Build history of the part. All positions in model axes, mm. Face numbers are marked on the shaded views. A direction names the side the tool comes from. Give positions to 0.01 mm unless a question says otherwise; leave off trailing zeros. Write each loop counter-clockwise with the first axis right and the second up, starting at its lowest first coordinate (ties: lowest second). Pieces come first, ordered by that corner, then holes. Notation, with made-up numbers: (1.25, 7) - (13.25, 7) arc R27 cw to (13.25, 43) - close; hole circle Ø11 at (-32, 48). An arc over 180 degrees is marked (long way). Use one line per item in the form item = value. Start each with the question number.
from build123d import *

# Parameters (mm, degrees)
F1_DEPTH = 6.35
F2_W     = 6
F2_H     = 6
F3_DEPTH = 6.35


# Not quite as in the source:
# - a length typed as a fraction of an inch, garbled in the dataset ("3 / 203.2 mm" for 3/8 in), is restored


with BuildPart() as f1:
    # F0 (on Front) → F1 (new body)
    with BuildSketch(Plane.XZ):
        with BuildLine():
            ThreePointArc((9.85, 6.4062469512), (11.2649900133, 3.3410327745), (11.75, 0))
            ThreePointArc((11.75, 0), (11.2649900133, -3.3410327745), (9.85, -6.4062469512))
            Line((9.85, -6.4062469512), (9.85, -13.5476935306))
            ThreePointArc((9.85, -13.5476935306), (14.9256490646, -7.6018089952), (16.75, 0))
            ThreePointArc((16.75, 0), (14.9256490646, 7.6018089952), (9.85, 13.5476935306))
            Line((9.85, 13.5476935306), (9.85, 6.4062469512))
        make_face()
        with BuildLine():
            ThreePointArc((-9.85, 6.4062469512), (0, 11.75), (9.85, 6.4062469512))
            Line((9.85, 6.4062469512), (9.85, 13.5476935306))
            ThreePointArc((9.85, 13.5476935306), (0, 16.75), (-9.85, 13.5476935306))
            Line((-9.85, 13.5476935306), (-9.85, 6.4062469512))
        make_face()
        with BuildLine():
            Line((9.85, -13.5476935306), (9.85, -6.4062469512))
            ThreePointArc((9.85, -6.4062469512), (0, -11.75), (-9.85, -6.4062469512))
            Line((-9.85, -6.4062469512), (-9.85, -13.5476935306))
            ThreePointArc((-9.85, -13.5476935306), (0, -16.75), (9.85, -13.5476935306))
        make_face()
        with BuildLine():
            ThreePointArc((-9.85, -6.4062469512), (-11.75, 0), (-9.85, 6.4062469512))
            Line((-9.85, 6.4062469512), (-9.85, 13.5476935306))
            ThreePointArc((-9.85, 13.5476935306), (-16.75, 0), (-9.85, -13.5476935306))
            Line((-9.85, -13.5476935306), (-9.85, -6.4062469512))
        make_face()
        with BuildLine():
            ThreePointArc((-9.85, 13.5476935306), (0, 16.75), (9.85, 13.5476935306))
            Line((9.85, 13.5476935306), (9.85, 30.31089))
            Line((9.85, 30.31089), (-9.85, 30.31089))
            Line((-9.85, 30.31089), (-9.85, 13.5476935306))
        make_face()
        with BuildLine():
            Line((9.85, -30.31089), (9.85, -13.5476935306))
            ThreePointArc((9.85, -13.5476935306), (0, -16.75), (-9.85, -13.5476935306))
            Line((-9.85, -13.5476935306), (-9.85, -30.31089))
            Line((-9.85, -30.31089), (9.85, -30.31089))
        make_face()
    extrude(amount=F1_DEPTH)

    # F2 (on face) → F3 (join)
    with BuildSketch(Plane.XZ.offset(6.35)):
        with Locations((-6.85, 33.31089)):
            Rectangle(F2_W, F2_H)
        with Locations((6.85, 33.31089)):
            Rectangle(F2_W, F2_H)
        with Locations((-6.85, -33.31089)):
            Rectangle(F2_W, F2_H)
        with Locations((6.85, -33.31089)):
            Rectangle(F2_W, F2_H)
    extrude(amount=-F3_DEPTH)


solid = f1.part
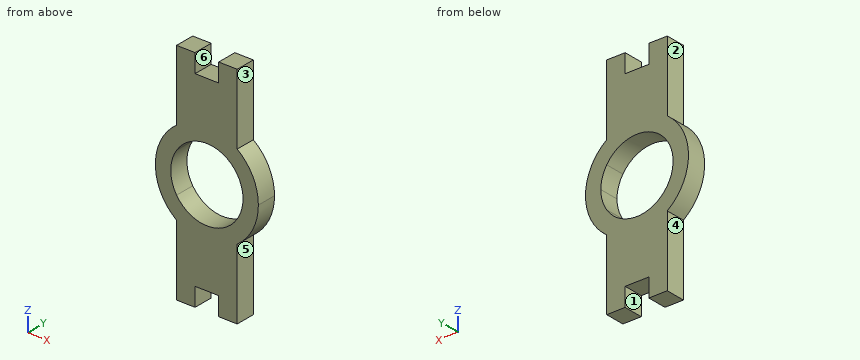
(1) Cut at D-D, the plane z = 28.5. Give the cut face in (x, y), then the cut area to 3 significant figures.
(2) Cut at A-A, the plane y = -1.25. Give the cut face in (x, z).
(3) Two-plate mould, pull along X, no slides. Class the marked faces 4, 5 and 6: +X half, -X half, draft (parallel to the pull), parting line (faces both ways), or undercut.
(4) Cut at B-B, the plane x = -5.5. Give the cut face in (y, z).
(5) Pin check, flat tips, straight feed: pin 1 Ø3 at (x, y) = (0.5, -3) entering from -Z; pin 2 Ø3 at (x, y) = (-1, -3.5) entering from +Z; pin 3 Ø3 at (x, y) = (12, -1) entering from -Z. Stop position of each tip, or through.
(6) Which spindle directions (+Z, -Z, +X, -X, +Y, -Y) get a long thin tool onto all of the face, cutting with end or side? Do the marked faces 1, 2 and 3. Say none if no direction does.
(7) Cut at C-C, the plane z = 8.5. Give the cut face in (x, y).
(8) Wall check: line 1 (Z direction, x = 2, y = -4.75); line 2 (Z direction, x = -9, y = -1); line 3 (X direction, y = -4.5, z = -1.5). Give the ranges that are in metal, low to high. Write a range as from..to.
Solution:
q1.outline = (-9.85, -6.35) - (9.85, -6.35) - (9.85, 0) - (-9.85, 0) - close
q1.area = 125 mm2
q2.outline = (-9.85, -36.31) - (-3.85, -36.31) - (-3.85, -30.31) - (3.85, -30.31) - (3.85, -36.31) - (9.85, -36.31) - (9.85, -13.55) arc R16.75 ccw to (9.85, 13.55) - (9.85, 36.31) - (3.85, 36.31) - (3.85, 30.31) - (-3.85, 30.31) - (-3.85, 36.31) - (-9.85, 36.31) - (-9.85, 13.55) arc R16.75 ccw to (-9.85, -13.55) - close; hole circle Ø23.5 at (0, 0)
q3.face_4 = -X half
q3.face_5 = +X half
q3.face_6 = undercut
q4.outline = (-6.35, -36.31) - (0, -36.31) - (0, -10.38) - (-6.35, -10.38) - close; (-6.35, 10.38) - (0, 10.38) - (0, 36.31) - (-6.35, 36.31) - close
q5.pin_1 = -30.31
q5.pin_2 = 30.31
q5.pin_3 = -13.05
q6.face_1 = -Z, +Y, -Y
q6.face_2 = +Z, -X, +Y, -Y
q6.face_3 = +Z, +X, +Y, -Y
q7.outline = (-14.43, -6.35) - (-8.11, -6.35) - (-8.11, 0) - (-14.43, 0) - close; (8.11, -6.35) - (14.43, -6.35) - (14.43, 0) - (8.11, 0) - close
q8.line_1 = -30.31..-11.58, 11.58..30.31
q8.line_2 = -36.31..-7.55, 7.55..36.31
q8.line_3 = -16.68..-11.65, 11.65..16.68
